from build123d import *
from build123d.topology import SkipClean

# Parameters (mm, degrees)
CROQUIS1_W              = 28
CROQUIS1_H              = 8
CROQUIS1_R              = 1.85
SALIENTE_EXTRUIR1_DEPTH = 7.5
SALIENTE_EXTRUIR2_DEPTH = 28
CROQUIS4_R              = 1.85
CORTAR_EXTRUIR1_DEPTH   = 20.416487839
CROQUIS5_R              = 3
CORTAR_EXTRUIR2_DEPTH   = 3.5
CORTAR_EXTRUIR3_DEPTH   = 25.899799196
CROQUIS7_R              = 3.5
CORTAR_EXTRUIR4_DEPTH   = 1.5
CROQUIS8_R              = 2.15
CORTAR_EXTRUIR5_DEPTH   = 5


with BuildPart() as part:
    # Croquis1 → Saliente-Extruir1 (new body)
    with BuildSketch(Plane(origin=(0, 0, 0), x_dir=(1, 0, 0), z_dir=(0, 1, 0))):
        Rectangle(CROQUIS1_W, CROQUIS1_H)
        with Locations(Location((-5.31, 0, 0), (0, 0, 270))):
            Circle(CROQUIS1_R, mode=Mode.SUBTRACT)
        with Locations(Location((4.69, 0, 0), (0, 0, 270))):
            Circle(CROQUIS1_R, mode=Mode.SUBTRACT)
    extrude(amount=SALIENTE_EXTRUIR1_DEPTH)

    # Croquis3 → Saliente-Extruir2 (add, through all)
    with BuildSketch(Plane.ZY.offset(14)):
        Polygon((-4.242640687, 0), (4.242640687, 0), (9, -4.757359313), (9, -10), (3.25, -10), (3.25, -8), (6, -8), (6, -6), (3, -3), (-3, -3), (-6, -6), (-6, -8), (-3.25, -8), (-3.25, -10), (-9, -10), (-9, -4.757359313), align=None)
    extrude(amount=-SALIENTE_EXTRUIR2_DEPTH)

    # Croquis4 → Cortar-Extruir1 (cut, through all)
    with SkipClean():  # the faces are left unmerged after this step: merging them gives an invalid solid
        with BuildSketch(Plane(origin=(0, 0, 0), x_dir=(1, 0, 0), z_dir=(0, 1, 0))):
            with Locations(Location((4.69, 0, 0), (0, 0, 90))):
                Circle(CROQUIS4_R)
            with Locations(Location((-5.31, 0, 0), (0, 0, 90))):
                Circle(CROQUIS4_R)
        extrude(amount=-CORTAR_EXTRUIR1_DEPTH, mode=Mode.SUBTRACT)

    # Croquis5 → Cortar-Extruir2 (cut)
    with BuildSketch(Plane.XZ.offset(3)):
        with Locations(Location((-5.31, 0, 0), (0, 0, 270))):
            Circle(CROQUIS5_R)
        with Locations(Location((4.69, 0, 0), (0, 0, 270))):
            Circle(CROQUIS5_R)
    extrude(amount=-CORTAR_EXTRUIR2_DEPTH, mode=Mode.SUBTRACT)

    # Croquis6 → Cortar-Extruir3 (cut, through all)
    with BuildSketch(Plane.XY.offset(9)):
        with BuildLine():
            ThreePointArc((-1.748852427, -4.757359313), (-0.378932969, -7.361829693), (1.9, -5.5))
            ThreePointArc((1.9, -5.5), (1.861829693, -5.121067031), (1.748852427, -4.757359313))
            Line((1.748852427, -4.757359313), (-1.748852427, -4.757359313))
        make_face()
        with BuildLine():
            Line((-1.748852427, -4.757359313), (1.748852427, -4.757359313))
            ThreePointArc((1.748852427, -4.757359313), (0, -3.6), (-1.748852427, -4.757359313))
        make_face()
    extrude(amount=-CORTAR_EXTRUIR3_DEPTH, mode=Mode.SUBTRACT)

    # Croquis7 → Cortar-Extruir4 (cut)
    with BuildSketch(Plane.XY.offset(9)):
        with Locations((0, -5.5)):
            Circle(CROQUIS7_R)
    extrude(amount=-CORTAR_EXTRUIR4_DEPTH, mode=Mode.SUBTRACT)

    # Croquis8 → Cortar-Extruir5 (cut)
    with BuildSketch(Plane.XY.offset(7.5)):
        with Locations((0, -5.5)):
            Circle(CROQUIS8_R)
    extrude(amount=-CORTAR_EXTRUIR5_DEPTH, mode=Mode.SUBTRACT)


solid = part.part
Build history of the part. All positions in model axes, mm. A direction names the side the tool comes from. Coordinates: 2 decimals unless noted, no trailing zeros. Order: outer loops, then holes, each group sorted by start corner. A loop starts at its lowest first (then second) coordinate and runs counter-clockwise, first axis right, second up. Notation, with made-up numbers: (-33, 77) - (16, 77) arc R25 ccw to (16, 91) - close; hole circle Ø2 at (4, -8.5). An arc over 180 degrees is marked (long way). Put each result on its own line as item: value.
1. Saw through at A-A (z = 0). Write the cut outline in (x, y).
Answer sheet:
outline: (-14, -3) - (-8.31, -3) - (-8.31, 0.5) - (-7.16, 0.5) - (-7.16, 7.5) - (-14, 7.5) - close; (-3.46, 0.5) - (-2.31, 0.5) - (-2.31, -3) - (1.69, -3) - (1.69, 0.5) - (2.84, 0.5) - (2.84, 7.5) - (-3.46, 7.5) - close; (6.54, 0.5) - (7.69, 0.5) - (7.69, -3) - (14, -3) - (14, 7.5) - (6.54, 7.5) - close
2. Probe line 1 along Z through (x, y) = (5.75, -7); line 2 along Z through (x, y) = (4.69, 3.5); line 3 along X through (y, z) = (-5.5, 8.45). List the from-to ranges inside material, lowest first. Write a range as [from, to].
Answer sheet:
line 1: z = [-9, -6], [6, 9]
line 2: z = [-4, -1.85], [1.85, 4]
line 3: x = [-14, -3.5], [3.5, 14]
3. Saw through at B-B (y = 4.75). Write the cut outline in (x, z).
Answer sheet:
outline: (-14, -4) - (14, -4) - (14, 4) - (-14, 4) - close; hole circle Ø3.7 at (-5.31, 0); hole circle Ø3.7 at (4.69, 0)
4. Tool access for faces 5 (the face through (0, -3, 0)), 6 (the face through (0, -8, 7.5)), 7 (the face through (0, 4, 4)), 8 (the face through (0, -8, -5)): list every direction of +Z, -Z, +X, -X, +Y, -Y with a clear straight run to the whole face (end or side of a thin tool).
Answer sheet:
face 5: +X, -X, -Y
face 6: +Z
face 7: +Z, +X, -X, +Y
face 8: +X, -X
5. Saw through at D-D (x = -6). Write the cut outline in (y, z).
Answer sheet:
outline: (-10, -9) - (-4.76, -9) - (0, -4.24) - (0, -4) - (7.5, -4) - (7.5, -1.72) - (0.5, -1.72) - (0.5, -2.92) - (-3, -2.92) - (-3, -3) - (-6, -6) - (-8, -6) - (-8, -3.25) - (-10, -3.25) - close; (-10, 3.25) - (-8, 3.25) - (-8, 6) - (-6, 6) - (-3, 3) - (-3, 2.92) - (0.5, 2.92) - (0.5, 1.72) - (7.5, 1.72) - (7.5, 4) - (0, 4) - (0, 4.24) - (-4.76, 9) - (-10, 9) - close
6. Pull direction Z, two halves, no side cores. Call faces 1 (the face through (10, -3, 0)), 2 (the face through (-0.2, -2.41, -6.65)), 3 (the face through (-14, -1, 0)), 4 (the face through (5, 0.5, -2)): pulls with the +Z half, pulls with the -Z half, needs draft (parallel to the pull), parting line crosses it, or undercut.
Answer sheet:
face 1: undercut
face 2: pulls with the -Z half
face 3: needs draft
face 4: undercut
7. Saw through at C-C (x = 9.5). Write the cut outline in (y, z), and give its area (3 significant figures).
Answer sheet:
outline: (-10, -9) - (-4.76, -9) - (0, -4.24) - (0, -4) - (7.5, -4) - (7.5, 4) - (0, 4) - (0, 4.24) - (-4.76, 9) - (-10, 9) - (-10, 3.25) - (-8, 3.25) - (-8, 6) - (-6, 6) - (-3, 3) - (-3, -3) - (-6, -6) - (-8, -6) - (-8, -3.25) - (-10, -3.25) - close
area: 153 mm^2
8. Drop flat-ended pins along their axis: P1, Ø3, axis at x = -4, z = 1, coming from the -Y side; P2, Ø2, axis at x = -1, y = 2.5, coming from the -Z side; P3, Ø4, axis at x = 0, y = -3, coming from the -Z side; P4, Ø3.5, axis at x = 4.69, z = 0, coming from the +Y side. Give the stop position or say it passes through.
Answer sheet:
P1: stops at y = -3
P2: stops at z = -4
P3: stops at z = -8.57
P4: passes through
